Source: CAD feature listing. Evaluate the final solid. Frame: model axes, mm. A direction names the side the tool comes from. Give positions to 0.01 mm unless a question says otherwise; leave off trailing zeros. Order: outer loops, then holes, each group sorted by start corner. A loop starts at its lowest first (then second) coordinate and runs counter-clockwise, first axis right, second up.
from build123d import *

# Parameters (mm, degrees)
SKETCH1_W                      = 240
SKETCH1_H                      = 300
BASE_FLANGE1_DEPTH             = 5
EDGE_FLANGE1_STRIP_W           = 21.4732
EDGE_FLANGE1_STRIP_H           = 5
EDGE_FLANGE1_STRIP_CUT_DEPTH   = 240
EDGE_FLANGE1_STRIP_2_W         = 21.4732
EDGE_FLANGE1_STRIP_2_H         = 5
EDGE_FLANGE1_STRIP_CUT_2_DEPTH = 240
EDGE_FLANGE1_DEPTH             = 240
EDGE_FLANGE1_BEND_DEPTH        = 240
CUT_EXTRUDE1_DEPTH             = 331.395217883
CUT_EXTRUDE1_DEPTH_BACK        = 331.395217883
SKETCH12_R                     = 7
SKETCH13_R                     = 42.5
SKETCH13_R_2                   = 9
CUT_EXTRUDE3_DEPTH             = 10


# Sheet-metal steps are written as plain solids
with BuildPart() as part:
    # Sketch1 → Base-Flange1 (new body)
    with BuildSketch(Plane(origin=(0, 0, 0), x_dir=(1, 0, 0), z_dir=(0, 1, 0))):
        Rectangle(SKETCH1_W, SKETCH1_H)
    extrude(amount=-BASE_FLANGE1_DEPTH)

    # Edge-Flange1 strip (across the edge) → Edge-Flange1 strip cut (cut)
    with BuildSketch(Plane(origin=(-120, -5, -150), x_dir=(0, 0, 1), z_dir=(1, 0, 0))):
        with Locations((-5, -2.5)):
            Rectangle(EDGE_FLANGE1_STRIP_W, EDGE_FLANGE1_STRIP_H)
    extrude(amount=EDGE_FLANGE1_STRIP_CUT_DEPTH, mode=Mode.SUBTRACT)

    # Edge-Flange1 strip 2 (across the edge) → Edge-Flange1 strip cut 2 (cut)
    with BuildSketch(Plane(origin=(120, -5, 150), x_dir=(0, 0, -1), z_dir=(-1, 0, 0))):
        with Locations((-5, -2.5)):
            Rectangle(EDGE_FLANGE1_STRIP_2_W, EDGE_FLANGE1_STRIP_2_H)
    extrude(amount=EDGE_FLANGE1_STRIP_CUT_2_DEPTH, mode=Mode.SUBTRACT)

    # Edge-Flange1 section (across the edge) → Edge-Flange1 (add)
    with BuildSketch(Plane(origin=(-120, -5, -150), x_dir=(0, 0, 1), z_dir=(1, 0, 0))):
        with BuildLine():
            Line((0, 0.7366), (0, 64))
            Line((0, 64), (5, 64))
            Line((5, 64), (5, 0.7366))
            ThreePointArc((5, 0.7366), (5.215745145, 0.215745145), (5.7366, 0))
            Line((5.7366, 0), (5.7366, -5))
            ThreePointArc((5.7366, -5), (1.680211239, -3.319788761), (0, 0.7366))
        make_face()
    extrude(amount=EDGE_FLANGE1_DEPTH)

    # Edge-Flange1 section 2 (across the edge) → Edge-Flange1 bend (add)
    with BuildSketch(Plane(origin=(120, -5, 150), x_dir=(0, 0, -1), z_dir=(-1, 0, 0))):
        with BuildLine():
            Line((0, 0.7366), (0, 64))
            Line((0, 64), (5, 64))
            Line((5, 64), (5, 0.7366))
            ThreePointArc((5, 0.7366), (5.215745145, 0.215745145), (5.7366, 0))
            Line((5.7366, 0), (5.7366, -5))
            ThreePointArc((5.7366, -5), (1.680211239, -3.319788761), (0, 0.7366))
        make_face()
    extrude(amount=EDGE_FLANGE1_BEND_DEPTH)

    # Sketch12 → Cut-Extrude1 (cut, two sides: drawn at the far end of the back side and taken through both)
    with BuildSketch(Plane(origin=(0, 0, -150), x_dir=(-1, 0, 0), z_dir=(0, 0, -1)).offset(-CUT_EXTRUDE1_DEPTH_BACK)):
        with Locations(Location((100, -49, 0), (0, 0, 90))):
            Circle(SKETCH12_R)
        with Locations(Location((-100, -49, 0), (0, 0, 90))):
            Circle(SKETCH12_R)
    extrude(amount=CUT_EXTRUDE1_DEPTH + CUT_EXTRUDE1_DEPTH_BACK, mode=Mode.SUBTRACT)

    # Sketch13 → Cut-Extrude3 (cut)
    with BuildSketch(Plane(origin=(0, 0, 0), x_dir=(1, 0, 0), z_dir=(0, 1, 0))):
        with Locations(Location((0, 0, 0), (0, 0, 270))):
            Circle(SKETCH13_R)
        with Locations(Location((79.5, 79.5, 0), (0, 0, 270))):
            Circle(SKETCH13_R_2)
        with Locations(Location((-79.5, 79.5, 0), (0, 0, 270))):
            Circle(SKETCH13_R_2)
        with Locations(Location((-79.5, -79.5, 0), (0, 0, 270))):
            Circle(SKETCH13_R_2)
        with Locations(Location((79.5, -79.5, 0), (0, 0, 270))):
            Circle(SKETCH13_R_2)
    extrude(amount=-CUT_EXTRUDE3_DEPTH, mode=Mode.SUBTRACT)


solid = part.part
1) Pull-direction query (Z, two-part tool) for faces 3 (the face through (106.94, -49.91, 147.54)), 4 (the face through (2, -37, 150)), 5 (the face through (71.515, -2.465, 83.653)); classes: +Z half, -Z half, draft (parallel to the pull), parting line (faces both ways), or undercut.
Checks:
face 3: draft
face 4: +Z half
face 5: undercut
2) First-contact query: pin 1 Ø1 at (x, z) = (-61, -115.5) entering from -Y. Flat tip, straight axial feed; report the tip coordinate or a pass-through.
Checks:
pin 1: stops at y = -5
3) Reachability of faces 1 (the face through (-28, 0, -34)), 2 (the face through (2, -38, 145)) from +Z, -Z, +X, -X, +Y, -Y: full face, straight path, thin tool, end or side. Return the list, or none.
Checks:
face 1: +Z, -Z, +X, -X, +Y
face 2: +X, -X, -Y
4) Section query D-D on y = -49. Output: boundary loops of the cut face in (x, z), and give its area (3 significant figures).
Checks:
outline: (-120, -150) - (-107, -150) - (-107, -145) - (-120, -145) - close; (-120, 145) - (-107, 145) - (-107, 150) - (-120, 150) - close; (-93, -150) - (93, -150) - (93, -145) - (-93, -145) - close; (-93, 145) - (93, 145) - (93, 150) - (-93, 150) - close; (107, -150) - (120, -150) - (120, -145) - (107, -145) - close; (107, 145) - (120, 145) - (120, 150) - (107, 150) - close
area: 2,120 mm2
5) Section query B-B on z = 79.5. Output: boundary loops of the cut face in (x, y).
Checks:
outline: (-120, -5) - (-88.5, -5) - (-88.5, 0) - (-120, 0) - close; (-70.5, -5) - (70.5, -5) - (70.5, 0) - (-70.5, 0) - close; (88.5, -5) - (120, -5) - (120, 0) - (88.5, 0) - close
6) Ray query, L1, parallel to X at y = -1, z = -79; L2, parallel to Z at x = 62.5, y = -40; L3, parallel to Y at x = -109, z = -82. Return the intervals inside material, ascending.
Checks:
L1: x = -120 to -88.49, -70.51 to 70.51, 88.49 to 120
L2: z = -150 to -145, 145 to 150
L3: y = -5 to 0
7) Section query A-A on y = -63.5. Output: boundary loops of the cut face in (x, z), and give its area (3 significant figures).
Checks:
outline: (-120, -150) - (120, -150) - (120, -145) - (-120, -145) - close; (-120, 145) - (120, 145) - (120, 150) - (-120, 150) - close
area: 2,400 mm2
8) Section query C-C on x = 100. Output: boundary loops of the cut face in (y, z), and give its area (3 significant figures).
Checks:
outline: (-69, -150) - (-56, -150) - (-56, -145) - (-69, -145) - close; (-69, 145) - (-56, 145) - (-56, 150) - (-69, 150) - close; (-42, -150) - (-5.74, -150) arc R5.74 ccw to (0, -144.26) - (0, 144.26) arc R5.74 ccw to (-5.74, 150) - (-42, 150) - (-42, 145) - (-5.74, 145) arc R0.74 cw to (-5, 144.26) - (-5, -144.26) arc R0.74 cw to (-5.74, -145) - (-42, -145) - close
area: 1,990 mm2
